Geometry: final body of the model. Coordinates: model frame, mm. A direction names the side the tool comes from. Give positions to 0.01 mm unless a question says otherwise; leave off trailing zeros. Order: outer loops, then holes, each group sorted by start corner. A loop starts at its lowest first (then second) coordinate and runs counter-clockwise, first axis right, second up. Notation, with made-up numbers: (56, 2.25) - (102, 2.25) arc R35 cw to (102, 36.25) - close; hole circle Ø7 at (19.5, -18). An arc over 180 degrees is marked (long way). Write item = value, one per line. Start each with the question number.
from build123d import *

# Parameters (mm, degrees)
SKETCH1_W           = 100
SKETCH1_H           = 120
SKETCH1_R           = 30
BOSS_EXTRUDE1_DEPTH = 40
SKETCH2_R           = 3.5
CUT_EXTRUDE1_DEPTH  = 15
CUT_EXTRUDE2_START  = -15
SKETCH3_R           = 3.5
CUT_EXTRUDE2_DEPTH  = 15


with BuildPart() as part:
    # Sketch1 → Boss-Extrude1 (new body)
    with BuildSketch(Plane.XY):
        with Locations((15.48649625, -14.939759036)):
            Rectangle(SKETCH1_W, SKETCH1_H)
        with Locations((15.48649625, -14.939759036)):
            Circle(SKETCH1_R, mode=Mode.SUBTRACT)
    extrude(amount=BOSS_EXTRUDE1_DEPTH)

    # Sketch2 → Cut-Extrude1 (cut)
    with BuildSketch(Plane.ZY.offset(34.51350375)):
        with Locations(Location((20, -14.939759036, 0), (0, 0, 270))):
            Circle(SKETCH2_R)
    extrude(amount=-CUT_EXTRUDE1_DEPTH, mode=Mode.SUBTRACT)

    # Sketch3 → Cut-Extrude2 (cut)
    with BuildSketch(Plane(origin=(65.48649625, 0, 0), x_dir=(0, 0, -1), z_dir=(1, 0, 0)).offset(CUT_EXTRUDE2_START)):
        with Locations(Location((-20, -14.939759036, 0), (0, 0, 270))):
            Circle(SKETCH3_R)
    extrude(amount=CUT_EXTRUDE2_DEPTH, mode=Mode.SUBTRACT)


solid = part.part
Q1. Contact query for flat-ended pins moving along their axis: pin 1 (4 mm diameter, centred on y = -14.94, z = 20, fed in from -X); pin 2 (6 mm diameter, centred on x = 16.5, y = 27.5, fed in from -Z); pin 3 (3.5 mm diameter, centred on y = -15.5, z = 21, fed in from +X). Output: stop coordinate, or through.
Q2. Section B-B, the plane y = -20. Return the cut outline in (x, z), then the cut area to 3 significant figures.
Q3. Pull-direction query (Y, two-part tool) for faces 4 (the cylindrical face through (-6.62, 5.34, 19.72)), 5 (the flat face through (65.486, -16, 24)), 6 (the flat face through (15, -74.94, 20)); classes: +Y half, -Y half, draft (parallel to the pull), parting line (faces both ways), or undercut.
Q4. Section A-A, the plane x = 29. Return the cut outline in (y, z), then the cut area to 3 significant figures.
Q5. Material intervals for line 1 along Y through (x, z) = (55, 20); line 2 along X through (y, z) = (-14, 36); line 3 along X through (y, z) = (-38, 38), sorted ascending. Write a range as from..to.
Q6. Section D-D, the plane z = 20. Return the cut outline in (x, y).
Q7. Set-up query: faces 1 (the flat face through (-19.514, -15, 20)), 2 (the cylindrical face through (57.88, -14.48, 16.53)), 3 (the flat face through (-34.514, -16, 24)). Return all of +Z, -Z, +X, -X, +Y, -Y with unobstructed straight access to the full face (end or side cutting, diameter ignored); none if empty.
Q8. Section C-C, the plane z = 26. Return the cut outline in (x, y), then the cut area to 3 significant figures.
The answers:
q1.pin_1 = -19.51
q1.pin_2 = 0
q1.pin_3 = 50.49
q2.outline = (-34.51, 0) - (-14.08, 0) - (-14.08, 40) - (-34.51, 40) - close; (45.06, 0) - (65.49, 0) - (65.49, 40) - (45.06, 40) - close
q2.area = 1,630 mm²
q3.face_4 = undercut
q3.face_5 = draft
q3.face_6 = -Y half
q4.outline = (-74.94, 0) - (-41.72, 0) - (-41.72, 40) - (-74.94, 40) - close; (11.84, 0) - (45.06, 0) - (45.06, 40) - (11.84, 40) - close
q4.area = 2,660 mm²
q5.line_1 = -74.94..-18.44, -11.44..45.06
q5.line_2 = -34.51..-14.5, 45.47..65.49
q5.line_3 = -34.51..-3.7, 34.68..65.49
q6.outline = (-34.51, -74.94) - (65.49, -74.94) - (65.49, -18.44) - (50.49, -18.44) - (50.49, -11.44) - (65.49, -11.44) - (65.49, 45.06) - (-34.51, 45.06) - (-34.51, -11.44) - (-19.51, -11.44) - (-19.51, -18.44) - (-34.51, -18.44) - close; hole circle Ø60 at (15.49, -14.94)
q7.face_1 = -X
q7.face_2 = +X
q7.face_3 = +Z, -Z, -X, +Y, -Y
q8.outline = (-34.51, -74.94) - (65.49, -74.94) - (65.49, 45.06) - (-34.51, 45.06) - close; hole circle Ø60 at (15.49, -14.94)
q8.area = 9,170 mm²
